Can you work these out from the drawing? Everything is in mm from the part's minimum corner. A direction names the side the tool comes from. Give positions to 0.01 mm unless a question says otherwise; leave off trailing zeros. Order: outer loops, then holes, each group sorted by start corner. A loop starts at its lowest first (then second) coordinate and runs counter-clockwise, first axis right, second up. Notation, with made-up numbers: M 77,35.5 L 123,35.5 A15 cw 123,60.5 Z; hole C 77,-13 d7. An arc over 180 degrees is marked long. Answer as a JSON object with one key per item and string values.
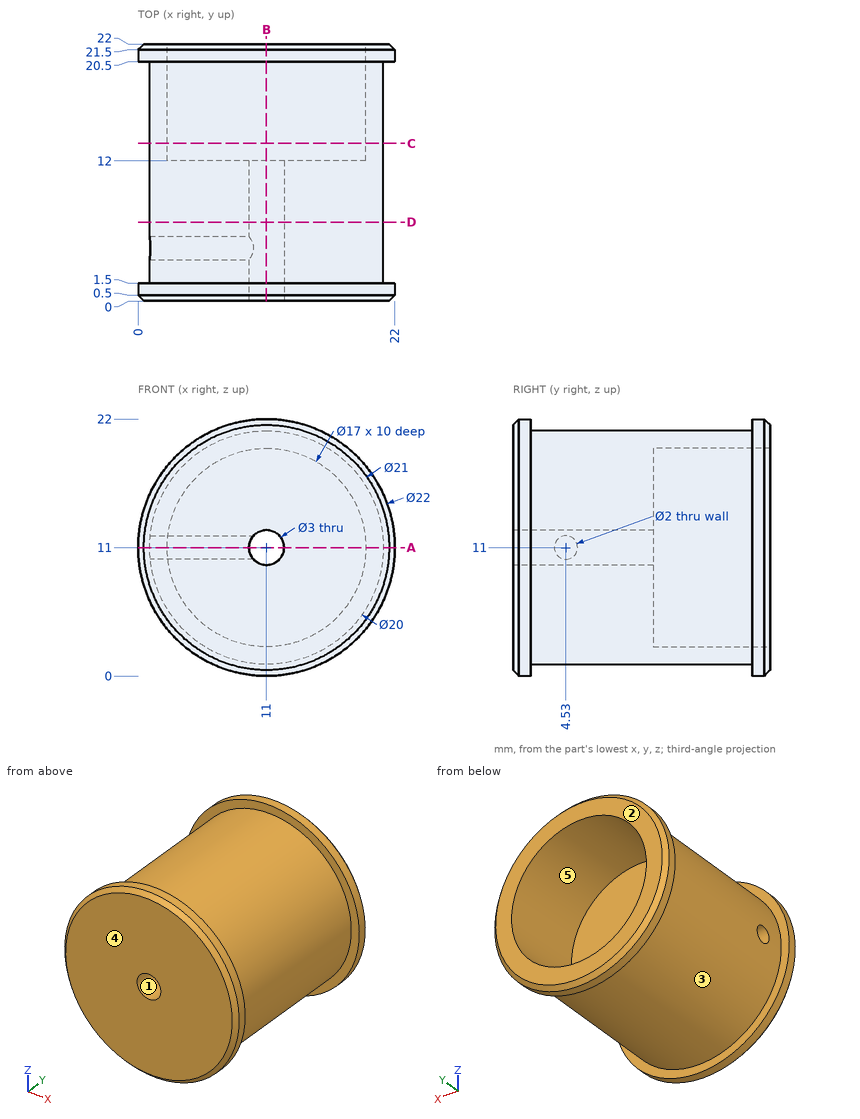
1) Thinking about a two-plate mould opening in Z: for the marked faces 1, 2 and 3, which applies, pulls with the +Z half, pulls with the -Z half, needs draft (parallel to the pull), parting line crosses it, or undercut?
Results found:
{"face 1": "undercut", "face 2": "needs draft", "face 3": "parting line crosses it"}
2) I want a section at C-C on y = 13.5. Write out the boundary of the cut face in (x, z).
Results found:
{"outline": "C 11,11 d20; hole C 11,11 d17"}
3) I want a section at D-D on y = 6.75. Write out the boundary of the cut face in (x, z).
Results found:
{"outline": "C 11,11 d20; hole C 11,11 d3"}
4) I'm going to push flat-ended pins straight in: pin 1 Ø12 at (x, y) = (17.5, 17) entering from +Z; pin 2 Ø12 at (y, z) = (18, 3) entering from +X; pin 3 Ø2.5 at (y, z) = (4.53, 11) entering from -X. Where does each tip first touch, or does it pass through?
Results found:
{"pin 1": "stops at z = 21.88", "pin 2": "stops at x = 21.7", "pin 3": "stops at x = 1"}
5) I need wall thicknesses on L1, parallel to Y at x = 18, z = 18.25; L2, parallel to Y at x = 5.5, z = 11; L3, parallel to X at y = 15, z = 11. Which ranges of each line are inside material? Lowest first, please.
Results found:
{"L1": "y = 0 to 1.5, 20.5 to 22", "L2": "y = 0 to 3.53, 5.53 to 12", "L3": "x = 1 to 2.5, 19.5 to 21"}
6) I want a section at A-A on z = 11. Write out the boundary of the cut face in (x, y).
Results found:
{"outline": "M 0,0.5 L 0.5,0 L 9.5,0 L 9.5,3.53 L 1,3.53 L 1,1.5 L 0,1.5 Z; M 0,20.5 L 1,20.5 L 1,5.53 L 9.5,5.53 L 9.5,12 L 2.5,12 L 2.5,22 L 0.5,22 L 0,21.5 Z; M 12.5,0 L 21.5,0 L 22,0.5 L 22,1.5 L 21,1.5 L 21,20.5 L 22,20.5 L 22,21.5 L 21.5,22 L 19.5,22 L 19.5,12 L 12.5,12 Z"}
7) I want a section at B-B on x = 11. Write out the boundary of the cut face in (y, z), and give its area (4 significant figures).
Results found:
{"outline": "M 0,0.5 L 0.5,0 L 1.5,0 L 1.5,1 L 20.5,1 L 20.5,0 L 21.5,0 L 22,0.5 L 22,2.5 L 12,2.5 L 12,9.5 L 0,9.5 Z; M 0,12.5 L 12,12.5 L 12,19.5 L 22,19.5 L 22,21.5 L 21.5,22 L 20.5,22 L 20.5,21 L 1.5,21 L 1.5,22 L 0.5,22 L 0,21.5 Z", "area": "239.5 mm²"}
8) For the marked faces 4 and 5, which set-ups out of +Z, -Z, +X, -X, +Y, -Y let a thin tool reach every point of the face, with its end or its side?
Results found:
{"face 4": "+Z, -Z, +X, -X, -Y", "face 5": "+Y"}
